```python
from build123d import *

# Parameters (mm, degrees)
BASE_FLANGE2_DEPTH = 825.5
SKETCH1_R          = 3.175
SKETCH1_R_2        = 2.413
SKETCH1_R_3        = 4.7625
SKETCH1_R_4        = 34.925
CUT_EXTRUDE3_DEPTH = 859.694710551


# Sheet-metal steps are written as plain solids
with BuildPart() as part:
    # Sketch3 → Base-Flange2 (new body)
    with BuildSketch(Plane.XY):
        with BuildLine():
            Line((3.175, 233.4895), (25.4, 233.4895))
            Line((25.4, 233.4895), (25.4, 235.077))
            Line((25.4, 235.077), (3.175, 235.077))
            ThreePointArc((3.175, 235.077), (0.92993597, 234.14706403), (0, 231.902))
            Line((0, 231.902), (0, 0))
            ThreePointArc((0, 0), (0.92993597, -2.24506403), (3.175, -3.175))
            Line((3.175, -3.175), (7.9375, -3.175))
            Line((7.9375, -3.175), (7.9375, -1.5875))
            Line((7.9375, -1.5875), (3.175, -1.5875))
            ThreePointArc((3.175, -1.5875), (2.052467985, -1.122532015), (1.5875, 0))
            Line((1.5875, 0), (1.5875, 231.902))
            ThreePointArc((1.5875, 231.902), (2.052467985, 233.024532015), (3.175, 233.4895))
        make_face()
    extrude(amount=-BASE_FLANGE2_DEPTH)

    # Sketch1 → Cut-Extrude3 (cut, through all)
    with BuildSketch(Plane(origin=(0, 0, 0), x_dir=(0, 0, -1), z_dir=(1, 0, 0))):
        with Locations(Location((516.509, 31.75, 0), (0, 0, 90))):
            Circle(SKETCH1_R)
        with Locations(Location((308.991, 31.75, 0), (0, 0, 90))):
            Circle(SKETCH1_R)
        with Locations(Location((103.492550911, 60.630923565, 0), (0, 0, 90))):
            Circle(SKETCH1_R)
        with Locations(Location((722.007449089, 60.630923565, 0), (0, 0, 90))):
            Circle(SKETCH1_R)
        with Locations(Location((412.75, 6.35, 0), (0, 0, 90))):
            Circle(SKETCH1_R_2)
        with Locations(Location((412.75, 88.9, 0), (0, 0, 90))):
            Circle(SKETCH1_R_2)
        with Locations(Location((622.478249316, 6.35, 0), (0, 0, 90))):
            Circle(SKETCH1_R_2)
        with Locations(Location((612.465522577, 88.9, 0), (0, 0, 90))):
            Circle(SKETCH1_R_2)
        with Locations(Location((203.021750684, 6.35, 0), (0, 0, 90))):
            Circle(SKETCH1_R_2)
        with Locations(Location((101.978503418, 46.225723918, 0), (0, 0, 90))):
            Circle(SKETCH1_R)
        with Locations(Location((723.521496582, 46.225723918, 0), (0, 0, 90))):
            Circle(SKETCH1_R)
        with Locations(Location((213.034477423, 88.9, 0), (0, 0, 90))):
            Circle(SKETCH1_R_2)
        with Locations(Location((510.45745, 97.70745, 0), (0, 0, 90))):
            Circle(SKETCH1_R_3)
        with Locations(Location((480.14255, 97.70745, 0), (0, 0, 90))):
            Circle(SKETCH1_R_3)
        with Locations(Location((480.14255, 67.39255, 0), (0, 0, 90))):
            Circle(SKETCH1_R_3)
        with Locations(Location((510.45745, 67.39255, 0), (0, 0, 90))):
            Circle(SKETCH1_R_3)
        with Locations(Location((345.35745, 97.70745, 0), (0, 0, 90))):
            Circle(SKETCH1_R_3)
        with Locations(Location((315.04255, 97.70745, 0), (0, 0, 90))):
            Circle(SKETCH1_R_3)
        with Locations(Location((345.35745, 67.39255, 0), (0, 0, 90))):
            Circle(SKETCH1_R_3)
        with Locations(Location((315.04255, 67.39255, 0), (0, 0, 90))):
            Circle(SKETCH1_R_3)
        with Locations(Location((330.2, 179.961124202, 0), (0, 0, 90))):
            Circle(SKETCH1_R_4)
        Polygon((775.673017562, -3.175), (825.5, 107.95), (825.5, -3.175), align=None)
        Polygon((0, 107.95), (0, -3.175), (49.826982438, -3.175), align=None)
    extrude(amount=CUT_EXTRUDE3_DEPTH, mode=Mode.SUBTRACT)


solid = part.part
```
Source: CAD feature listing. Evaluate the final solid. Frame: model axes, mm. A direction names the side the tool comes from. Round coordinates to 2 decimals unless told otherwise and drop trailing zeros. Loops run counter-clockwise (first coordinate to the right, second up) from the corner with the lowest first, then second, coordinate; pieces in that order, holes last. Notation, with made-up numbers: M 73,48.25 L 82,48.25 A26 ccw 82,63.25 Z; hole C -18.5,88 d3. An arc over 180 degrees is marked long. Put each result on its own line as item: value.
(1) Access query for faces 1 (the face through (14, 233.49, -407)), 2 (the face through (0, 118, -407)). Directions: +Z, -Z, +X, -X, +Y, -Y. A direction counts if a zero-diameter tool reaches every point of the face in a straight line with its end or side. Return the directions, or none.
Solutions:
face 1: +Z, -Z, +X
face 2: +Z, -Z, -X, +Y, -Y
(2) Section C-C, the plane x = 17.25. Return loops of the section in (y, z).
Solutions:
outline: M 233.49,-825.5 L 235.08,-825.5 L 235.08,0 L 233.49,0 Z
(3) Ray query, line 1 (Y direction, x = 4.5, z = -173.5) (1 decimal); line 2 (Z direction, x = 1, y = 6.35); line 3 (X direction, y = 126, z = -393). Return the intervals inside material, ascending. Write a range as [from, to].
Solutions:
line 1: [-3.2, -1.6], [233.5, 235.1]
line 2: [-779.94, -624.89], [-620.07, -415.16], [-410.34, -205.43], [-200.61, -45.56]
line 3: [0, 1.59]
(4) Pull-direction query (Y, two-part tool) for faces 3 (the face through (1.588, 114, -407)), 4 (the face through (1.01, 52.13, -25.03)), 5 (the face through (0.4, 171.8, 0)); classes: released by +Y, released by -Y, zero draft, split by the parting line, or undercut.
Solutions:
face 3: undercut
face 4: released by -Y
face 5: zero draft
(5) First-contact query: pin 1 (8.5 mm diameter, centred on y = 31.75, z = -516.509, fed in from +X); pin 2 (3 mm diameter, centred on y = 88.9, z = -213.03, fed in from +X). Flat tips, straight axial feed; report the tip coordinate or a pass-through.
Solutions:
pin 1: x = 1.59
pin 2: through
